The figure shows three views and two pictorial views of one solid part (mm, origin at its lowest corner). Answer the questions. A direction names the side the tool comes from. Round coordinates to 2 decimals unless told otherwise and drop trailing zeros. Order: outer loops, then holes, each group sorted by start corner. A loop starts at its lowest first (then second) coordinate and runs counter-clockwise, first axis right, second up. Notation, with made-up numbers: (41, -14) - (50, -14) arc R14 cw to (50, -9) - close; hole circle Ø9 at (-39.75, 57.25). An arc over 180 degrees is marked (long way). One line per item, written item: value. Start each with the question number.
1. Section A-A, the plane y = 2.5 is taken. Give the vertices of the cut face in (x, z), then the cut area to 3 significant figures.
2. Section D-D, the plane y = 8.75 is taken. Give the vertices of the cut face in (x, z) (1 decimal), then the cut area to 3 significant figures.
3. A tool of negligible diameter and unlimited length cuts with its end or side. For the marked faces 1, 2 and 3, from which of +Z, -Z, +X, -X, +Y, -Y can it reach the whole face along a straight path? Write none if from no direction.
4. Section B-B, the plane x = 29 is taken. Give the vertices of the cut face in (y, z).
5. For a pull along X with two mould halves and no side action, classify the marked faces 4, 5, 6 and 7 as released by +X, released by -X, zero draft, split by the parting line, or undercut.
6. Section C-C, the plane z = 26 is taken. Give the vertices of the cut face in (x, y), then the cut area to 3 significant figures.
7. Flat-ended cylindrical pins translate along their axes: P1, Ø2.5, axis at y = 6.5, z = 16.5, coming from the -X side; P2, Ø3, axis at y = 12, z = 20, coming from the -X side; P3, Ø12, axis at x = 40, z = 4, coming from the -Y side; P4, Ø3.5, axis at x = 33.5, z = 17, coming from the -Y side. Find the tip coordinate at first contact, or state that the pin passes through.
8. Straight lines are drawn through the part: line 1 (Y direction, x = 44.5, z = 3); line 2 (Y direction, x = 12, z = 15.25); line 3 (Z direction, x = 3.5, y = 1.5). For each, find the intervals that lie inside material, in ascending order.
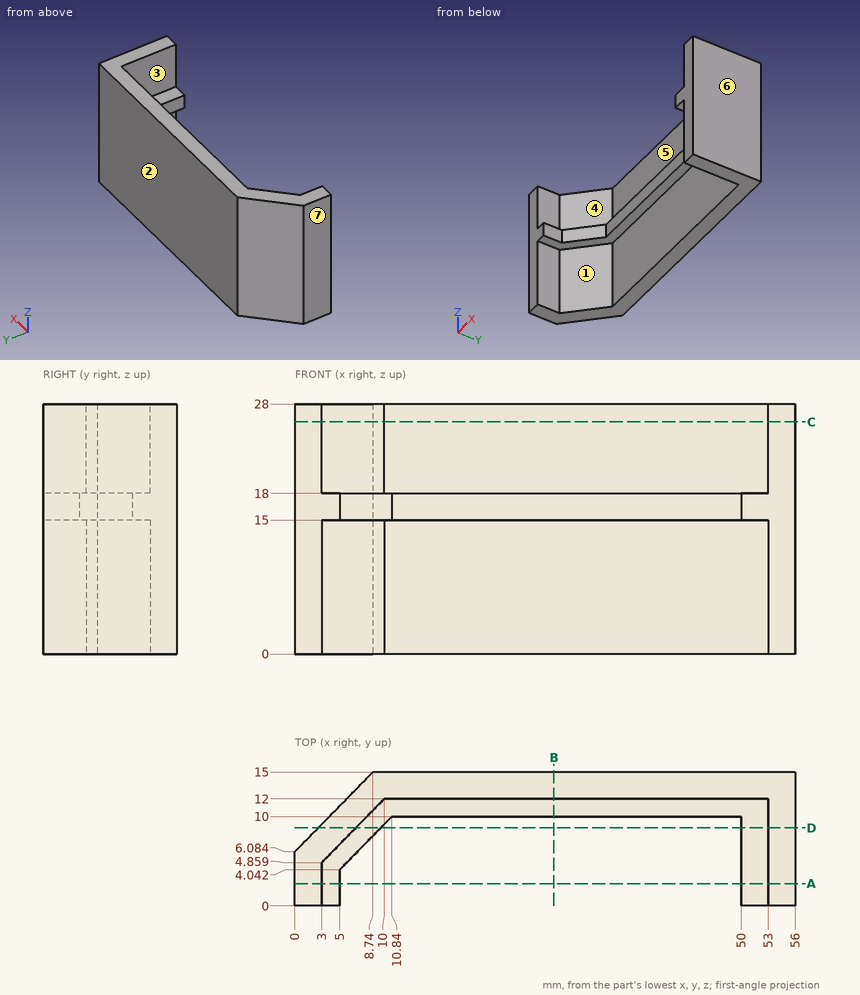
Answer list:
1. outline: (0, 0) - (3, 0) - (3, 15) - (5, 15) - (5, 18) - (3, 18) - (3, 28) - (0, 28) - close; (50, 15) - (53, 15) - (53, 0) - (56, 0) - (56, 28) - (53, 28) - (53, 18) - (50, 18) - close
1. area: 183 mm²
2. outline: (2.6, 0) - (6.8, 0) - (6.8, 15) - (9.6, 15) - (9.6, 18) - (6.8, 18) - (6.8, 28) - (2.6, 28) - close; (50, 15) - (53, 15) - (53, 0) - (56, 0) - (56, 28) - (53, 28) - (53, 18) - (50, 18) - close
2. area: 219 mm²
3. face 1: -Z, -Y
3. face 2: +Z, -Z, +X, -X, +Y
3. face 3: +Z, -Y
4. outline: (10, 15) - (12, 15) - (12, 0) - (15, 0) - (15, 28) - (12, 28) - (12, 18) - (10, 18) - close
5. face 4: undercut
5. face 5: undercut
5. face 6: released by +X
5. face 7: released by -X
6. outline: (0, 0) - (3, 0) - (3, 4.86) - (10, 12) - (53, 12) - (53, 0) - (56, 0) - (56, 15) - (8.74, 15) - (0, 6.08) - close
6. area: 226 mm²
7. P1: stops at x = 0
7. P2: stops at x = 4.33
7. P3: stops at y = 12
7. P4: stops at y = 10
8. line 1: y = 12 to 15
8. line 2: y = 10 to 15
8. line 3: z = 15 to 18
